The model under review builds one solid part; all positions refer to its coordinate system, in mm. A direction names the side the tool comes from. Coordinates: 2 decimals unless noted, no trailing zeros. Loops run counter-clockwise (first coordinate to the right, second up) from the corner with the lowest first, then second, coordinate; pieces in that order, holes last. Notation, with made-up numbers: M 23,75 L 50,75 A17 cw 50,98 Z; hole C 43,17 d7. An arc over 180 degrees is marked long. Write item = value, one per line. Start each with the question number.
Q1. We need section D-D on y = 10.5. Give the boundary of the cut face in (x, z).
Q2. Clearance check with flat-ended pins moving along their axes: pin 1 Ø2 at (x, z) = (7.5, -7) entering from +Y; pin 2 Ø0.9 at (x, z) = (5, -1) entering from +Y; pin 3 Ø3.5 at (x, z) = (8.7, 0) entering from -Y. State where each tip first meets the part, or that it passes through.
Q3. Mouldability with a two-part tool opening along Z and no side actions: class faces 4 (the face through (-2.97, 29.23, -3.99)), 5 (the face through (4.94, 29.23, -0.58)), 6 (the face through (3.969, 29.226, 2.976)) as released by +Z, released by -Z, zero draft, split by the parting line, or undercut.
Q4. Wall thickness on probe 1 along Z at (x, y) = (8.7, 5.65); probe 2 along X at (y, z) = (36.7, 0); probe 3 along Y at (x, z) = (5, -1.5): over which ranges is each line inside the solid? List them lowest first.
Q5. For faces 1 (the face through (-1.971, 29.226, 4.567)), 2 (the face through (10.732, 2.514, -0.843)), 3 (the face through (0, 36, 1)), list the 3-axis set-ups (+Z, -Z, +X, -X, +Y, -Y) from which the entire face can be reached by the end or side of a thin tool; tool diameter is ignored.
Q6. We need section A-A on y = 27. Give the boundary of the cut face in (x, z), and give its area (3 significant figures).
Q7. We need section B-B on x = -8.5. Give the boundary of the cut face in (y, z).
Q8. We need section C-C on z = -8.7. Give the boundary of the cut face in (x, y), and give its area (3 significant figures).
from build123d import *

# Parameters (mm, degrees)
SKETCH1_R            = 10.2
BOSS_EXTRUDE1_DEPTH  = 1.2
SKETCH3_R            = 5.5
BOSS_EXTRUDE2_DEPTH  = 22.8
SKETCH6_R            = 3.3
BOSS_EXTRUDE7_DEPTH  = 6.3
SKETCH7_R            = 2.2
CUT_EXTRUDE1_DEPTH   = 5.1
SKETCH8_R            = 1.1
CUT_EXTRUDE2_DEPTH   = 1.2
CIRPATTERN1_COUNT    = 4
SKETCH9_R            = 4.4
CUT_EXTRUDE3_DEPTH   = 22.8
SKETCH10_R           = 4.5
BOSS_EXTRUDE8_DEPTH  = 10.6
BOSS_EXTRUDE9_DEPTH  = 10.6
CIRPATTERN2_COUNT    = 12
SKETCH12_R           = 3.2
CUT_EXTRUDE4_DEPTH   = 10.6
SKETCH13_R           = 2.3
BOSS_EXTRUDE10_DEPTH = 3
SKETCH14_R           = 1
CUT_EXTRUDE5_DEPTH   = 3


with BuildPart() as part:
    # Sketch1 → Boss-Extrude1 (new body)
    with BuildSketch(Plane(origin=(0, 0, 0), x_dir=(1, 0, 0), z_dir=(0, 1, 0))):
        Circle(SKETCH1_R)
    extrude(amount=BOSS_EXTRUDE1_DEPTH)

    # Sketch3 → Boss-Extrude2 (add)
    with BuildSketch(Plane(origin=(0, 1.2, 0), x_dir=(1, 0, 0), z_dir=(0, 1, 0))):
        Circle(SKETCH3_R)
    extrude(amount=BOSS_EXTRUDE2_DEPTH)

    # Sketch6 → Boss-Extrude7 (add)
    with BuildSketch(Plane.XZ):
        with Locations((8.7, 0)):
            Circle(SKETCH6_R)
    boss_extrude7 = extrude(amount=-BOSS_EXTRUDE7_DEPTH)

    # Sketch7 → Cut-Extrude1 (cut)
    with BuildSketch(Plane.XZ):
        with Locations((8.7, 0)):
            Circle(SKETCH7_R)
    cut_extrude1 = extrude(amount=-CUT_EXTRUDE1_DEPTH, mode=Mode.SUBTRACT)

    # Sketch8 → Cut-Extrude2 (cut)
    with BuildSketch(Plane(origin=(0, 6.3, 0), x_dir=(1, 0, 0), z_dir=(0, 1, 0))):
        with Locations((8.7, 0)):
            Circle(SKETCH8_R)
    cut_extrude2 = extrude(amount=-CUT_EXTRUDE2_DEPTH, mode=Mode.SUBTRACT)

    # CirPattern1: Boss-Extrude7, Cut-Extrude1, Cut-Extrude2 ×4 about axis
    cirpattern1_axis = Axis((0, 0, 0), (0, 1, 0))
    for i in range(1, CIRPATTERN1_COUNT):
        add(boss_extrude7.rotate(cirpattern1_axis, i * 360 / CIRPATTERN1_COUNT))
        add(cut_extrude1.rotate(cirpattern1_axis, i * 360 / CIRPATTERN1_COUNT), mode=Mode.SUBTRACT)
        add(cut_extrude2.rotate(cirpattern1_axis, i * 360 / CIRPATTERN1_COUNT), mode=Mode.SUBTRACT)

    # Sketch9 → Cut-Extrude3 (cut)
    with BuildSketch(Plane(origin=(0, 0, 0), x_dir=(-1, 0, 0), z_dir=(0, -1, 0))):
        Circle(SKETCH9_R)
    extrude(amount=-CUT_EXTRUDE3_DEPTH, mode=Mode.SUBTRACT)

    # Sketch10 → Boss-Extrude8 (add)
    with BuildSketch(Plane(origin=(0, 24, 0), x_dir=(1, 0, 0), z_dir=(0, 1, 0))):
        Circle(SKETCH10_R)
    extrude(amount=BOSS_EXTRUDE8_DEPTH)

    # Sketch11 → Boss-Extrude9 (add)
    with BuildSketch(Plane(origin=(0, 24, 0), x_dir=(1, 0, 0), z_dir=(0, 1, 0))):
        Polygon((-1.2, 4.337049688), (1.2, 4.337049688), (0, 5.5), align=None)
    boss_extrude9 = extrude(amount=BOSS_EXTRUDE9_DEPTH)

    # CirPattern2: Boss-Extrude9 ×12 about axis
    cirpattern2_axis = Axis((0, 0, 0), (0, 1, 0))
    for i in range(1, CIRPATTERN2_COUNT):
        add(boss_extrude9.rotate(cirpattern2_axis, i * 360 / CIRPATTERN2_COUNT))

    # Sketch12 → Cut-Extrude4 (cut)
    with BuildSketch(Plane.XZ.offset(-22.8)):
        Circle(SKETCH12_R)
    extrude(amount=-CUT_EXTRUDE4_DEPTH, mode=Mode.SUBTRACT)

    # Sketch13 → Boss-Extrude10 (add)
    with BuildSketch(Plane(origin=(0, 34.6, 0), x_dir=(1, 0, 0), z_dir=(0, 1, 0))):
        Circle(SKETCH13_R)
    extrude(amount=BOSS_EXTRUDE10_DEPTH)

    # Sketch14 → Cut-Extrude5 (cut)
    with BuildSketch(Plane(origin=(0, 37.6, 0), x_dir=(1, 0, 0), z_dir=(0, 1, 0))):
        Circle(SKETCH14_R)
    extrude(amount=-CUT_EXTRUDE5_DEPTH, mode=Mode.SUBTRACT)


solid = part.part
Returned:
q1.outline = C 0,0 d11; hole C 0,0 d8.8
q2.pin_1 = 1.2
q2.pin_2 = 34.6
q2.pin_3 = 5.1
q3.face_4 = released by -Z
q3.face_5 = undercut
q3.face_6 = released by +Z
q4.probe_1 = -3.3 to -1.1, 1.1 to 3.3
q4.probe_2 = -2.3 to -1, 1 to 2.3
q4.probe_3 = 0 to 24
q5.face_1 = +Z, +Y
q5.face_2 = -Y
q5.face_3 = +Y
q6.outline = M -5.5,0 L -4.37,-1.17 L -4.76,-2.75 L -3.2,-3.2 L -2.75,-4.76 L -1.17,-4.37 L 0,-5.5 L 1.17,-4.37 L 2.75,-4.76 L 3.2,-3.2 L 4.76,-2.75 L 4.37,-1.17 L 5.5,0 L 4.37,1.17 L 4.76,2.75 L 3.2,3.2 L 2.75,4.76 L 1.17,4.37 L 0,5.5 L -1.17,4.37 L -2.75,4.76 L -3.2,3.2 L -4.76,2.75 L -4.37,1.17 Z; hole C 0,0 d6.4
q6.area = 45.0 mm^2
q7.outline = M 0,-5.64 L 1.2,-5.64 L 1.2,-3.29 L 6.3,-3.29 L 6.3,-1.08 L 5.1,-1.08 L 5.1,-2.19 L 0,-2.19 Z; M 0,2.19 L 5.1,2.19 L 5.1,1.08 L 6.3,1.08 L 6.3,3.29 L 1.2,3.29 L 1.2,5.64 L 0,5.64 Z
q8.outline = M -5.32,0 L -2.2,0 L -2.2,5.1 L -1.1,5.1 L -1.1,6.3 L -3.3,6.3 L -3.3,1.2 L -5.32,1.2 Z; M 1.1,5.1 L 2.2,5.1 L 2.2,0 L 5.32,0 L 5.32,1.2 L 3.3,1.2 L 3.3,6.3 L 1.1,6.3 Z
q8.area = 21.4 mm^2
